The listing builds one solid part. Answer for the finished solid, in the listing's coordinates (mm). A direction names the side the tool comes from. Give positions to 0.01 mm unless a question says otherwise; leave off trailing zeros. Write each loop counter-clockwise with the first axis right and the second up, starting at its lowest first coordinate (ties: lowest second). Pieces come first, ordered by that corner, then holes. Notation, with made-up numbers: (24, 66.25) -> (73, 66.25) arc R20 ccw to (73, 94.25) -> close; hole circle Ø2 at (-22, 74). An arc over 180 degrees is marked (long way). Put each result on its own line as item: value. Start each with the question number.
1) A cutting plane is placed at B-B (z = -7). Write down the section's boundary in (x, y), then the cut area to 3 significant figures.
2) For faces 1 (the cylindrical face through (-0.03, 1.27, -10.75)), 2 (the flat face through (6.6, 37.77, -2.51)), 3 (the flat face through (2, 36.5, 3)), determine the directions among +Z, -Z, +X, -X, +Y, -Y from which every point of the face is accessible in a straight line to the end or side of a thin tool.
3) A cutting plane is placed at C-C (z = 0). Give the number of separate pieces and of enclosed holes in the cut face, then the cut area to 3 significant figures.
4) A cutting plane is placed at A-A (x = 0). Write down the section's boundary in (y, z).
5) Flat-ended cylindrical pins translate along their axes: pin 1 Ø3 at (y, z) = (21, 2) entering from -X; pin 2 Ø2 at (x, z) = (0, -9) entering from -Y; pin 3 Ø5 at (y, z) = (34.5, -4.5) entering from -X; pin 4 Ø6 at (y, z) = (7.5, -4.5) entering from +X. Find the tip coordinate at first contact, or state that the pin passes through.
6) For a pull along Z with two mould halves and no side action, classify faces 4 (the flat face through (6.6, 1.23, -2.51)), 5 (the flat face through (0, 39, 3)), 6 (the cylindrical face through (-0.03, 37.73, -10.75)) as released by +Z, released by -Z, zero draft, split by the parting line, or undercut.
7) A cutting plane is placed at D-D (x = -9.5). Write down the section's boundary in (y, z).
8) Find the intervals of material crossed by line 1 along Z through (x, y) = (0, 1.7); line 2 along Y through (x, z) = (-3.25, 8.75); line 3 along X through (y, z) = (37.25, -9), in increasing order. Write a range as from..to.
from build123d import *

# Parameters (mm, degrees)
SKETCH1_R           = 12
SKETCH1_R_2         = 1.75
BOSS_EXTRUDE1_DEPTH = 2.5
CUT_EXTRUDE3_DEPTH  = 2.5
SKETCH4_R           = 1.25
CUT_EXTRUDE4_DEPTH  = 5
SKETCH2_R           = 3
SKETCH2_R_2         = 1.75
BOSS_EXTRUDE2_DEPTH = 17


with BuildPart() as part:
    # Sketch1 → Boss-Extrude1 (new body)
    with BuildSketch(Plane(origin=(0, 0, 0), x_dir=(1, 0, 0), z_dir=(0, 1, 0))):
        Circle(SKETCH1_R)
        Circle(SKETCH1_R_2, mode=Mode.SUBTRACT)
    extrude(amount=BOSS_EXTRUDE1_DEPTH)

    # Sketch3 → Cut-Extrude3 (cut)
    with BuildSketch(Plane.XZ):
        Polygon((-5.161329605, 1.721273866), (-8.071331697, 3.318997608), (-10.910002092, 1.597723742), (-10.838670395, -1.721273866), (-7.928668303, -3.318997608), (-5.089997908, -1.597723742), align=None)
        Polygon((5.161329605, -1.721273866), (8.071331697, -3.318997608), (10.910002092, -1.597723742), (10.838670395, 1.721273866), (7.928668303, 3.318997608), (5.089997908, 1.597723742), align=None)
    extrude(amount=-CUT_EXTRUDE3_DEPTH, mode=Mode.SUBTRACT)

    # Sketch4 → Cut-Extrude4 (cut)
    with BuildSketch(Plane(origin=(0, 2.5, 0), x_dir=(1, 0, 0), z_dir=(0, 1, 0))):
        with Locations((0, 9)):
            Circle(SKETCH4_R)
        with Locations((0, 12)):
            Circle(SKETCH4_R)
    extrude(amount=-CUT_EXTRUDE4_DEPTH, mode=Mode.SUBTRACT)

    # Sketch2 → Boss-Extrude2 (add)
    with BuildSketch(Plane(origin=(0, 2.5, 0), x_dir=(1, 0, 0), z_dir=(0, 1, 0))):
        Circle(SKETCH2_R)
        Circle(SKETCH2_R_2, mode=Mode.SUBTRACT)
    extrude(amount=BOSS_EXTRUDE2_DEPTH)

    # Mirror7: part across plane


with BuildPart() as part_1:
    add(part.part)
    add(part.part.mirror(Plane.ZX.offset(19.5)))


solid = part_1.part
Reply:
1. outline: (-9.75, 0) -> (9.75, 0) -> (9.75, 2.5) -> (-9.75, 2.5) -> close; (-9.75, 36.5) -> (9.75, 36.5) -> (9.75, 39) -> (-9.75, 39) -> close
1. area: 97.5 mm2
2. face 1: -Z, +Y, -Y
2. face 2: +Y, -Y
2. face 3: none
3. separate pieces: 6
3. enclosed holes: 0
3. area: 130 mm2
4. outline: (0, -10.75) -> (2.5, -10.75) -> (2.5, -10.25) -> (0, -10.25) -> close; (0, -7.75) -> (2.5, -7.75) -> (2.5, -3) -> (36.5, -3) -> (36.5, -7.75) -> (39, -7.75) -> (39, -1.75) -> (0, -1.75) -> close; (0, 1.75) -> (39, 1.75) -> (39, 12) -> (36.5, 12) -> (36.5, 3) -> (2.5, 3) -> (2.5, 12) -> (0, 12) -> close; (36.5, -10.75) -> (39, -10.75) -> (39, -10.25) -> (36.5, -10.25) -> close
5. pin 1: stops at x = -2.96
5. pin 2: passes through
5. pin 3: stops at x = -11.62
5. pin 4: stops at x = 2.6
6. face 4: undercut
6. face 5: zero draft
6. face 6: released by -Z
7. outline: (0, -7.33) -> (2.5, -7.33) -> (2.5, -2.46) -> (0, -2.46) -> close; (0, 2.45) -> (2.5, 2.45) -> (2.5, 7.33) -> (0, 7.33) -> close; (36.5, -7.33) -> (39, -7.33) -> (39, -2.46) -> (36.5, -2.46) -> close; (36.5, 2.45) -> (39, 2.45) -> (39, 7.33) -> (36.5, 7.33) -> close
8. line 1: z = -10.75..-10.25, -7.75..-1.75, 1.75..12
8. line 2: y = 0..2.5, 36.5..39
8. line 3: x = -7.94..-1.25, 1.25..7.94
